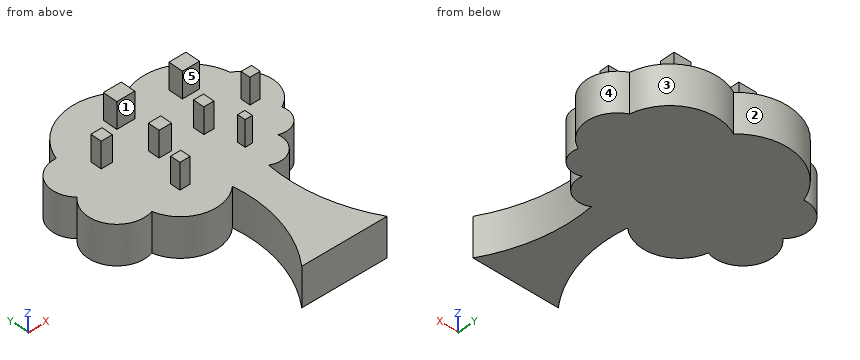
from build123d import *

# Parameters (mm, degrees)
F1_DEPTH = 19.05
F2_W     = 4.956221
F2_H     = 4.832608
F2_W_2   = 6.044237
F2_H_2   = 5.597412
F2_W_3   = 4.906744
F2_H_3   = 5.397417
F2_W_4   = 8.298278
F2_H_4   = 7.053539
F2_W_5   = 8.713215
F2_W_6   = 5.397439
F2_H_5   = 5.397424
F2_W_7   = 3.502958
F2_H_6   = 3.859587
F2_W_8   = 5.006534
F2_H_7   = 4.553236
F3_DEPTH = 12.7


with BuildPart() as f1:
    # F0 (on Top) → F1 (new body)
    with BuildSketch(Plane.XY):
        with BuildLine():
            ThreePointArc((-8.71323, -20.953164), (-9.969081, -47.283156), (-21.57557, -70.950329))
            Line((-21.57557, -70.950329), (19.915849, -70.950329))
            ThreePointArc((19.915849, -70.950329), (10.252818, -46.867793), (8.920625, -20.953164))
            ThreePointArc((8.920625, -20.953164), (19.332917, -20.334627), (23.027718, -10.580301))
            ThreePointArc((23.027718, -10.580301), (32.298513, -9.043512), (34.852773, 0))
            ThreePointArc((34.852773, 0), (43.232597, 13.380993), (34.852773, 26.761986))
            ThreePointArc((34.852773, 26.761986), (21.73884, 44.102992), (0, 43.773465))
            ThreePointArc((0, 43.773465), (-24.771472, 50.65636), (-43.830308, 33.40061))
            ThreePointArc((-43.830308, 33.40061), (-56.08557, 26.187958), (-53.316519, 12.239978))
            ThreePointArc((-53.316519, 12.239978), (-56.12724, -5.430092), (-39.416879, -11.82504))
            ThreePointArc((-39.416879, -11.82504), (-26.680312, -25.185865), (-8.71323, -20.953164))
        make_face()
    extrude(amount=F1_DEPTH)

    # F2 (on face) → F3 (join)
    with BuildSketch(Plane.XY.offset(19.05)):
        with Locations((-21.390158, -7.391732)):
            Rectangle(F2_W, F2_H)
        with Locations((-13.875554, 11.341883)):
            Rectangle(F2_W_2, F2_H_2)
        with Locations((6.275192, 10.112039)):
            Rectangle(F2_W_3, F2_H_3)
        with Locations((16.181633, 30.911125)):
            Rectangle(F2_W_4, F2_H_4)
        with Locations((-12.447461, 34.230441)):
            Rectangle(F2_W_5, F2_H_4)
        with Locations((-33.469454, 20.78421)):
            Rectangle(F2_W_6, F2_H_5)
        with Locations((11.407079, -5.958605)):
            Rectangle(F2_W_7, F2_H_6)
        with Locations((29.765008, 10.771705)):
            Rectangle(F2_W_8, F2_H_7)
    extrude(amount=F3_DEPTH)


solid = f1.part
Geometry: final body of the model. Coordinates: model frame, mm. Face numbers are marked on the shaded views. A direction names the side the tool comes from. Coordinates: 2 decimals unless noted, no trailing zeros. Loops run counter-clockwise (first coordinate to the right, second up) from the corner with the lowest first, then second, coordinate; pieces in that order, holes last. Notation, with made-up numbers: (35, -6) - (77, -6) arc R16 ccw to (77, 4) - close; hole circle Ø1 at (0.5, 2). An arc over 180 degrees is marked (long way). Put each result on its own line as item: value. Start each with the question number.
Q1. Set-up query: the marked faces 1 and 2. Return all of +Z, -Z, +X, -X, +Y, -Y with unobstructed straight access to the full face (end or side cutting, diameter ignored); none if empty.
Q2. Pin query (flat end, axial travel): pin 1 Ø12 at (y, z) = (-46, 23) entering from -X; pin 2 Ø2.5 at (x, z) = (15, 25) entering from -Y; pin 3 Ø3 at (y, z) = (11.5, 27) entering from +X. Return the tip coordinate at first contact, or that it passes through.
Q3. Pull-direction query (X, two-part tool) for the marked faces 3, 4 and 5; classes: released by +X, released by -X, zero draft, split by the parting line, or undercut.
Q4. Line query: line 1 (Z direction, x = 6.5, y = 15); line 2 (Y direction, x = -19, z = 5.5); line 3 (Y direction, x = -32, z = 23). Output: solid intervals per line, ascending.
Q5. Cut plane A-A, the plane z = 28. Give the number of separate pieces and of enclosed holes in the cut face, and give its area (3 significant figures).
Q6. Cut plane D-D, the plane y = 21. Return loops of the section in (x, z).
Q7. Cut plane C-C, the plane z = 9. Return loops of the section in (x, y).
Q8. Cut plane B-B, the plane x = -14.5. Return loops of the section in (y, z), and give its area (3 significant figures).
Filled sheet:
1. face 1: +Z, -X
1. face 2: +Z, -Z, +Y
2. pin 1: x = -10.89
2. pin 2: y = 27.38
2. pin 3: x = 32.27
3. face 3: undercut
3. face 4: released by +X
3. face 5: zero draft
4. line 1: 0 to 19.05
4. line 2: -70.95 to -67.39, -25.8 to 51.37
4. line 3: 18.09 to 23.48
5. separate pieces: 8
5. enclosed holes: 0
5. area: 270 mm²
6. outline: (-57.16, 0) - (41.13, 0) - (41.13, 19.05) - (-30.77, 19.05) - (-30.77, 31.75) - (-36.17, 31.75) - (-36.17, 19.05) - (-57.16, 19.05) - close
7. outline: (-53.32, 12.24) arc R14.2 ccw to (-39.42, -11.83) arc R18.56 ccw to (-8.71, -20.95) arc R65.01 cw to (-21.58, -70.95) - (19.92, -70.95) arc R78.94 cw to (8.92, -20.95) arc R9.59 ccw to (23.03, -10.58) arc R8.77 ccw to (34.85, 0) arc R14.87 ccw to (34.85, 26.76) arc R24.04 ccw to (0, 43.77) arc R26.65 ccw to (-43.83, 33.4) arc R12.28 ccw to start
8. outline: (-70.95, 0) - (-59.59, 0) - (-59.59, 19.05) - (-70.95, 19.05) - close; (-24.63, 0) - (51.05, 0) - (51.05, 19.05) - (37.76, 19.05) - (37.76, 31.75) - (30.7, 31.75) - (30.7, 19.05) - (14.14, 19.05) - (14.14, 31.75) - (8.54, 31.75) - (8.54, 19.05) - (-24.63, 19.05) - close
8. area: 1,820 mm²
